```python
from build123d import *

# Parameters (mm, degrees)
SKETCH1_W           = 6
SKETCH1_H           = 6
BOSS_EXTRUDE1_DEPTH = 5
CUT_EXTRUDE4_DEPTH  = 12.5
CUT_EXTRUDE5_DEPTH  = 10
CUT_EXTRUDE6_DEPTH  = 10


with BuildPart() as part:
    # Sketch1 → Boss-Extrude1 (new body)
    with BuildSketch(Plane(origin=(0, 0, 0), x_dir=(1, 0, 0), z_dir=(0, 1, 0))):
        Rectangle(SKETCH1_W, SKETCH1_H)
    extrude(amount=BOSS_EXTRUDE1_DEPTH)

    # Sketch5 → Cut-Extrude4 (cut)
    with BuildSketch(Plane.XY.offset(3)):
        with BuildLine():
            Line((-3, 5), (-3, 2.5))
            ThreePointArc((-3, 2.5), (-1.952562419, 4.293074903), (0, 5))
            Line((0, 5), (-3, 5))
        make_face()
        with BuildLine():
            ThreePointArc((0, 5), (1.952562419, 4.293074903), (3, 2.5))
            Line((3, 2.5), (3, 5))
            Line((3, 5), (0, 5))
        make_face()
        with BuildLine():
            ThreePointArc((-3, 0), (0, 2), (3, 0))
            Line((3, 0), (-3, 0))
        make_face()
    extrude(amount=-CUT_EXTRUDE4_DEPTH, mode=Mode.SUBTRACT)

    # 3DSketch1 → Cut-Extrude5 (cut, along a direction that is not the sketch's normal)
    with BuildSketch(Plane(origin=(-3, 1, 3), x_dir=(0.5383808129093879, 0.7133433044036882, -0.4486506774244899), z_dir=(0.5775173034874745, -0.700038740615242, -0.4200232443691449))):
        Polygon((0, 0), (2.19164165, -1.922682209), (5.572263959, 0), (3.380622309, 1.922682209), align=None)
    extrude(amount=-CUT_EXTRUDE5_DEPTH, dir=(1, 0, 0), mode=Mode.SUBTRACT)

    # Sketch7 → Cut-Extrude6 (cut)
    with BuildSketch(Plane(origin=(0, 3.878630283, 2.32717817), x_dir=(1, 0, 0), z_dir=(0, -0.8574929257125444, -0.5144957554275263))):
        with BuildLine():
            Line((-0.390198698, -2.130837603), (0, -2.130837603))
            Line((0, -2.130837603), (0, 0.784638345))
            Line((0, 0.784638345), (-2.641413746, 0.784638345))
            add(Edge.make_bspline(
                [(-2.641413746, 0.784638345), (-1.886895872, -1.755586828), (-0.390198698, -2.130837603)],
                knots=[2.094371322, 2.094371322, 2.094371322, 3.013307074, 3.013307074, 3.013307074], degree=2, weights=[1, 0.896288606, 1]))
        make_face()
    extrude(amount=-CUT_EXTRUDE6_DEPTH, mode=Mode.SUBTRACT)


solid = part.part
```
For this review, take the finished solid that the model builds, in its own axes (mm). A direction names the side the tool comes from. Coordinates: 2 decimals unless noted, no trailing zeros. Loops run counter-clockwise (first coordinate to the right, second up) from the corner with the lowest first, then second, coordinate; pieces in that order, holes last. Notation, with made-up numbers: (89.25, 59) - (93.25, 59) arc R16 cw to (93.25, 83) - close; hole circle Ø7 at (23.25, 61.5). An arc over 180 degrees is marked (long way). Use one line per item in the form item = value. Start each with the question number.
1) For pin 1 (2.5 mm diameter, centred on x = -2, y = 3.5, fed in from +Z); pin 2 (1.2 mm diameter, centred on y = 4.5, z = 2, fed in from -X), all flat-tipped, find the tip position at first contact; note any pin that passes through.
2) To check wall thickness, follow probe 1 along Z at (x, y) = (-1.25, 4.4); probe 2 along X at (y, z) = (1.4, -0.3); probe 3 along X at (y, z) = (0.6, -1.35). State the ranges of each line that lie inside material, in increasing order. Write a range as from..to.
3) Take a section at D-D (x = -2.5). State the section outline as (y, z) points, plus the area to 3 significant figures.
4) For faces 1 (the face through (0, 4.5, 2.3)), 2 (the face through (1, 2, 3)), list the 3-axis set-ups (+Z, -Z, +X, -X, +Y, -Y) from which the entire face can be reached by the end or side of a thin tool; tool diameter is ignored.
5) Take a section at A-A (y = 0.9). State the section outline as (x, z) points.
6) Draft analysis for pull direction X (two halves, no side actions). For faces 3 (the face through (0, 3, -3)), 4 (the face through (3, 1, 0)), 5 (the face through (-3, 1, 0)), 6 (the face through (0, 2, 0)), state which applies: released by +X, released by -X, zero draft, split by the parting line, or undercut.
7) Take a section at B-B (z = -0.05). State the section outline as (x, y) points, plus the area to 3 significant figures.
8) Take a section at C-C (y = 4.4). State the section outline as (x, z) points, plus the area to 3 significant figures.
From the geometry:
q1.pin_1 = 2.91
q1.pin_2 = -0.33
q2.probe_1 = -3..0.5
q2.probe_2 = -3..-1.88, 1.88..3
q2.probe_3 = -3..-2.67, 2.67..3
q3.outline = (0.83, -3) - (3.7, -3) - (3.7, 0.5) - (2.91, 0.5) - (1.41, 3) - (0.83, 3) - close
q3.area = 13.4 mm2
q4.face_1 = +Z, -X, +Y
q4.face_2 = +Z, +X, -X, +Y, -Y
q5.outline = (-3, -3) - (-2.44, -3) - (-2.44, 3) - (-3, 3) - close; (2.44, -3) - (3, -3) - (3, 3) - (2.44, 3) - close
q6.face_3 = zero draft
q6.face_4 = released by +X
q6.face_5 = released by -X
q6.face_6 = undercut
q7.outline = (-3, 0) arc R3.25 cw to (3, 0) - (3, 2.5) arc R3.05 ccw to (-3, 2.5) - close
q7.area = 17.6 mm2
q8.outline = (-1.82, -3) - (1.82, -3) - (1.82, 3) - (0, 3) - (0, 1.46) - (-0.7, 0.5) - (-1.82, 0.5) - close
q8.area = 17.6 mm2
